Can you work these out from the model? Positions are in its coordinate system, mm. A direction names the side the tool comes from. Round coordinates to 2 decimals unless told otherwise and drop trailing zeros. Order: outer loops, then holes, each group sorted by start corner. A loop starts at its lowest first (then second) coordinate and runs counter-clockwise, first axis right, second up. Notation, with made-up numbers: (53.25, 63.5) - (67.25, 63.5) arc R12 cw to (67.25, 77.5) - close; hole circle Ø8 at (-2.75, -1.75). An arc over 180 degrees is marked (long way). Write item = value, one per line.
from build123d import *

# Parameters (mm, degrees)
SKETCH025_R     = 19
PAD012_DEPTH    = 61.5
SKETCH026_R     = 11
PAD013_DEPTH    = 10.5
SKETCH027_R     = 11
PAD014_DEPTH    = 8
SKETCH028_R     = 3.75
PAD015_DEPTH    = 2
SKETCH029_R     = 1
POCKET011_DEPTH = 2
CHAMFER002_SIZE = 0.5
SKETCH030_R     = 3.75
PAD016_DEPTH    = 2.1
SKETCH031_R     = 3.175
PAD017_DEPTH    = 20.18
POCKET012_DEPTH = 15.6
SKETCH033_R     = 1
POCKET013_DEPTH = 2
CHAMFER003_SIZE = 0.5


with BuildPart() as part:
    # Sketch025 → Pad012 (new body)
    with BuildSketch(Plane.XZ):
        Circle(SKETCH025_R)
    extrude(amount=-PAD012_DEPTH)

    # Sketch026 (on Face2 of Pad012) → Pad013 (join)
    with BuildSketch(Plane.XZ):
        Circle(SKETCH026_R)
    extrude(amount=PAD013_DEPTH)

    # Sketch027 (on Face3 of Pad013) → Pad014 (join)
    with BuildSketch(Plane(origin=(0, 61.5, 0), x_dir=(1, 0, 0), z_dir=(0, 1, 0))):
        Circle(SKETCH027_R)
    extrude(amount=PAD014_DEPTH)

    # Sketch028 (on Face7 of Pad014) → Pad015 (join)
    with BuildSketch(Plane(origin=(0, 69.5, 0), x_dir=(1, 0, 0), z_dir=(0, 1, 0))):
        Circle(SKETCH028_R)
    extrude(amount=PAD015_DEPTH)

    # Sketch029 (on Face9 of Pad015) → Pocket011 (cut)
    with BuildSketch(Plane(origin=(0, 71.5, 0), x_dir=(1, 0, 0), z_dir=(0, 1, 0))):
        Circle(SKETCH029_R)
    extrude(amount=-POCKET011_DEPTH, mode=Mode.SUBTRACT)

    # Chamfer002
    chamfer002_edges = [part.edges().sort_by_distance(p)[0] for p in [
        (-3.75, 71.5, 0),
        (-1, 71.5, 0),
    ]]
    chamfer(chamfer002_edges, length=CHAMFER002_SIZE)

    # Sketch030 (on Face13 of Chamfer002) → Pad016 (join)
    with BuildSketch(Plane.XZ.offset(10.5)):
        Circle(SKETCH030_R)
    extrude(amount=PAD016_DEPTH)

    # Sketch031 (on Face15 of Pad016) → Pad017 (join)
    with BuildSketch(Plane.XZ.offset(12.6)):
        Circle(SKETCH031_R)
    extrude(amount=PAD017_DEPTH)

    # Sketch032 (on Face17 of Pad017) → Pocket012 (cut)
    with BuildSketch(Plane.XZ.offset(32.78)):
        with BuildLine():
            Line((-1.898315, 2.545), (1.898315, 2.545))
            ThreePointArc((1.898315, 2.545), (0, 3.175), (-1.898315, 2.545))
        make_face()
    extrude(amount=-POCKET012_DEPTH, mode=Mode.SUBTRACT)

    # Sketch033 (on Face17 of Pocket012) → Pocket013 (cut)
    with BuildSketch(Plane.XZ.offset(32.78)):
        Circle(SKETCH033_R)
    extrude(amount=-POCKET013_DEPTH, mode=Mode.SUBTRACT)

    # Chamfer003
    chamfer003_edges = [part.edges().sort_by_distance(p)[0] for p in [
        (-1, -32.78, 0),
        (-1.423635, -32.78, -2.837937),
        (2.837937, -32.78, 1.423635),
    ]]
    chamfer(chamfer003_edges, length=CHAMFER003_SIZE)


with BuildPart() as part_1:
    # Body010 placement: moved
    add(part.part.moved(Location((0, 11, 0))))


solid = part_1.part
(1) If we section it at C-C (y = 29.5): Write out the boundary of the cut face in (x, z).
Computed:
outline = circle Ø38 at (0, 0)
(2) Thinking about a two-plate mould opening in X: for faces 1 (the face through (0, 80.5, 0)), 2 (the face through (8.767, 41.32, -16.856)), 3 (the face through (0.7, 82.5, -1.5)), which applies, +X half, -X half, draft (parallel to the pull), parting line (faces both ways), or undercut?
Computed:
face_1 = undercut
face_2 = parting line
face_3 = draft
(3) If we section it at A-A (z = -6): Write out the boundary of the cut face in (x, y), plus the area to 3 significant figures.
Computed:
outline = (-18.03, 11) - (-9.22, 11) - (-9.22, 0.5) - (9.22, 0.5) - (9.22, 11) - (18.03, 11) - (18.03, 72.5) - (9.22, 72.5) - (9.22, 80.5) - (-9.22, 80.5) - (-9.22, 72.5) - (-18.03, 72.5) - close
area = 2,560 mm^2
(4) If I drill on line 1 (Z direction, x = 0, y = 81); line 2 (Z direction, x = 0, y = -20) (3 decimals), over which ranges is the centre line in solid material (lowest first)? Write a range as from..to.
Computed:
line_1 = -3.75..-1, 1..3.75
line_2 = -3.175..-1, 1..2.545
(5) Will these pins go through, and if not, where does the flat tip stop? P1, Ø2.5, axis at x = 0, z = 0, coming from the +Y side; P2, Ø1.6, axis at x = 0, z = 0, coming from the +Y side; P3, Ø1.5, axis at y = 19.5, z = 5, coming from the -X side.
Computed:
P1 = 82.25
P2 = 80.5
P3 = -18.52
(6) If we section it at D-D (z = -12.5): Write out the boundary of the cut face in (x, y), plus the area to 3 significant figures.
Computed:
outline = (-14.31, 11) - (14.31, 11) - (14.31, 72.5) - (-14.31, 72.5) - close
area = 1,760 mm^2
(7) If we section it at B-B (x = -9): Write out the boundary of the cut face in (y, z).
Computed:
outline = (0.5, -6.32) - (11, -6.32) - (11, -16.73) - (72.5, -16.73) - (72.5, -6.32) - (80.5, -6.32) - (80.5, 6.32) - (72.5, 6.32) - (72.5, 16.73) - (11, 16.73) - (11, 6.32) - (0.5, 6.32) - close
(8) On a 3-axis mill with a long thin cutter (end or side, diameter ignored), from which of +Z, -Z, +X, -X, +Y, -Y can I reach the whole of each face in a straight line? I mean faces 4 (the face through (0, 0.5, -5)), 5 (the face through (0, -14, 2.545)), 6 (the face through (0, 80.5, 5)). Say none if no direction works.
Computed:
face_4 = -Y
face_5 = +Z, +X, -X, -Y
face_6 = +Y
